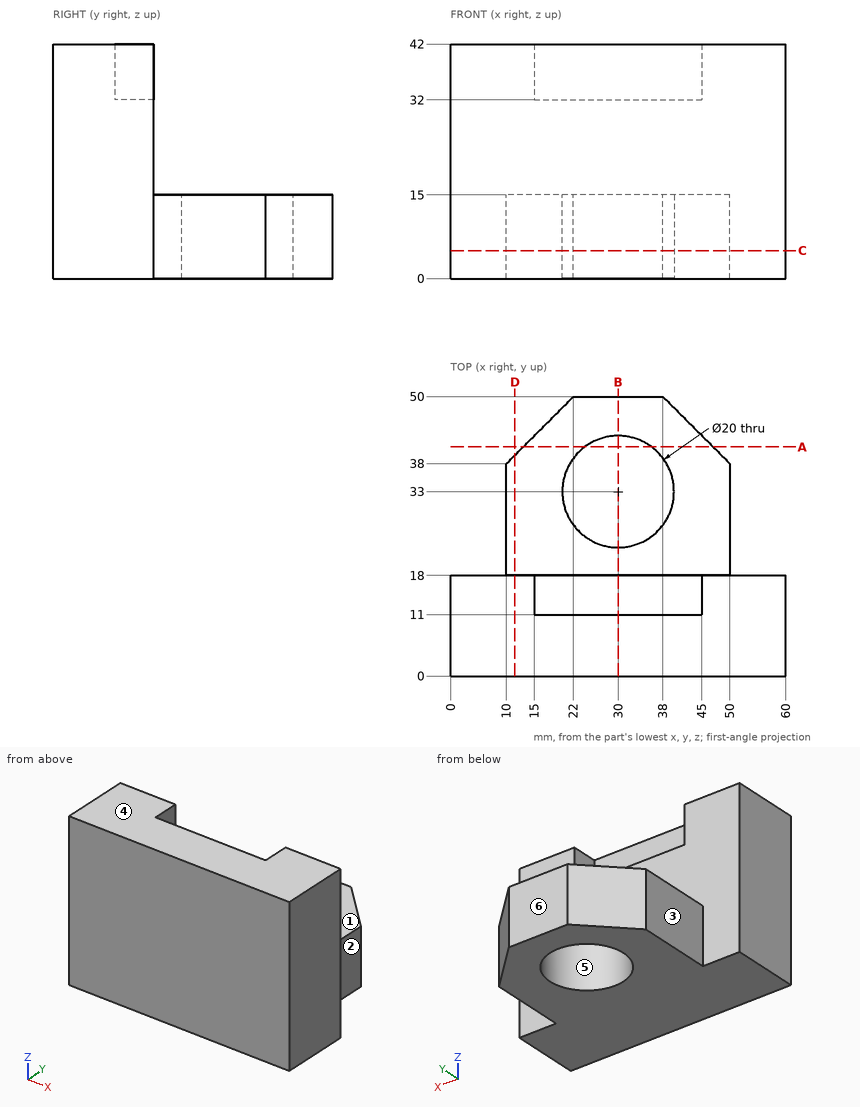
Can you work these out from the drawing? Everything is in mm from the part's minimum corner. A direction names the side the tool comes from. Round coordinates to 2 decimals unless told otherwise and drop trailing zeros. Loops run counter-clockwise (first coordinate to the right, second up) from the corner with the lowest first, then second, coordinate; pieces in that order, holes last. Notation, with made-up numbers: (-34, 9.5) - (-14, 9.5) arc R7 ccw to (-14, 17.5) - close; hole circle Ø9 at (27.5, 78). An arc over 180 degrees is marked (long way). Answer in a Markdown table with one row per item. Add a question column.
(1) If we section it at A-A (y = 41): Please give me the cut outline in (x, z), plus the area to 3 significant figures.
(2) I need wall thicknesses on line 1 along Y through (x, z) = (30, 9); line 2 along Z through (x, y) = (20.5, 12); line 3 along Y through (x, z) = (3, 39.5). Which ranges of each line are inside material? Lowest first, please.
(3) If we section it at D-D (x = 11.5): Please give me the cut outline in (y, z), plus the area to 3 significant figures.
(4) I'm going to push flat-ended pins straight in: pin 1 (11 mm diameter, centred on x = 31, z = 34.5, fed in from +Y); pin 2 (16.5 mm diameter, centred on y = 32, z = 11, fed in from +X); pin 3 (5.5 mm diameter, centred on x = 23, y = 14, fed in from +Z). Where does each tip first touch, or does it pass through?
(5) For the marked faces 1, 2 and 3, which set-ups out of +Z, -Z, +X, -X, +Y, -Y let a thin tool reach every point of the face, with its end or its side?
(6) If we mould it in two halves opening along Y, with no side actions, what happens to the marked faces 4, 5 and 6? For each: pulls with the +Y half, pulls with the -Y half, needs draft (parallel to the pull), parting line crosses it, or undercut.
(7) If we section it at C-C (z = 5): Please give me the cut outline in (x, y).
(8) If we section it at B-B (x = 30): Please give me the cut outline in (y, z).
Model answer:
| question | item | result |
|---|---|---|
| 1 | outline | (13, 0) - (24, 0) - (24, 15) - (13, 15) - close; (36, 0) - (47, 0) - (47, 15) - (36, 15) - close |
| 1 | area | 330 mm² |
| 2 | line 1 | y = 0 to 23, 43 to 50 |
| 2 | line 2 | z = 0 to 32 |
| 2 | line 3 | y = 0 to 18 |
| 3 | outline | (0, 0) - (39.5, 0) - (39.5, 15) - (18, 15) - (18, 42) - (0, 42) - close |
| 3 | area | 1,080 mm² |
| 4 | pin 1 | stops at y = 18 |
| 4 | pin 2 | stops at x = 50 |
| 4 | pin 3 | stops at z = 32 |
| 5 | face 1 | +Z, +X, -X, +Y |
| 5 | face 2 | +Z, -Z, +X, +Y |
| 5 | face 3 | +Z, -Z, -X, +Y |
| 6 | face 4 | needs draft |
| 6 | face 5 | undercut |
| 6 | face 6 | pulls with the +Y half |
| 7 | outline | (0, 0) - (60, 0) - (60, 18) - (50, 18) - (50, 38) - (38, 50) - (22, 50) - (10, 38) - (10, 18) - (0, 18) - close; hole circle Ø20 at (30, 33) |
| 8 | outline | (0, 0) - (23, 0) - (23, 15) - (18, 15) - (18, 32) - (11, 32) - (11, 42) - (0, 42) - close; (43, 0) - (50, 0) - (50, 15) - (43, 15) - close |
